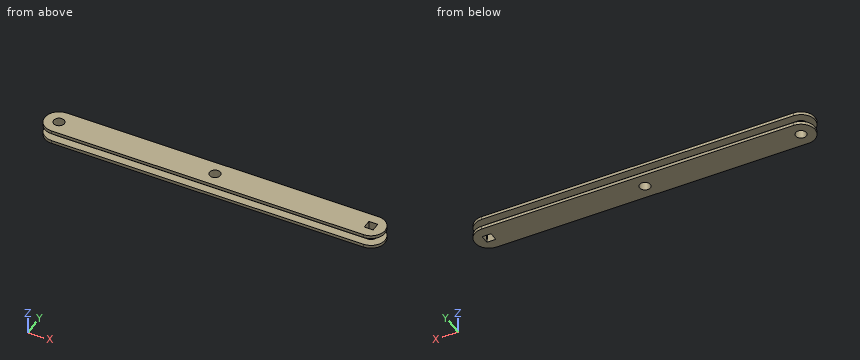
from build123d import *

# Parameters (mm, degrees)
ESQUISSE1_W             = 152.4
ESQUISSE1_H             = 12.7
BOSS_EXTRU_1_DEPTH      = 6.35
ESQUISSE2_W             = 3.967596046
ESQUISSE2_H             = 3.967596046
ESQUISSE2_W_2           = 3.367596046
ESQUISSE2_H_2           = 3.367596046
ESQUISSE2_W_3           = 3.167596046
ESQUISSE2_H_3           = 3.167596046
ESQUISSE2_R             = 2.38125
ENL_V_MAT_EXTRU_1_DEPTH = 154.060029074
SKETCH1_W               = 14.17076538
SKETCH1_H               = 3.495000122
CUT_REVOLVE1_ANGLE      = 180
SKETCH2_W               = 3.495000122
SKETCH2_H               = 3.683
CUT_EXTRUDE1_DEPTH      = 154.060029074
ESQUISSE2_3_W           = 3.367596046
ESQUISSE2_3_H           = 3.367596046
ESQUISSE2_3_W_2         = 3.167596046
ESQUISSE2_3_H_2         = 3.167596046
CUT_EXTRUDE2_DEPTH      = 154.060029074


with BuildPart() as part:
    # Esquisse1 → Boss.-Extru.1 (new body)
    with BuildSketch(Plane.XY):
        with Locations((-76.2, 6.35)):
            Rectangle(ESQUISSE1_W, ESQUISSE1_H)
    extrude(amount=-BOSS_EXTRU_1_DEPTH)

    # Esquisse2 → Enlèv. mat.-Extru.1 (cut, through all)
    # profile 1 of 8: a face of its own
    with BuildSketch(Plane.XY):
        with BuildLine():
            Line((0, 0), (0, 6.35))
            ThreePointArc((0, 6.35), (-1.859871939, 1.859871939), (-6.35, 0))
            Line((-6.35, 0), (0, 0))
        make_face()
    # profile 2 of 8: a face of its own
    with BuildSketch(Plane.XY):
        with BuildLine():
            Line((0, 12.7), (-6.35, 12.7))
            ThreePointArc((-6.35, 12.7), (-1.859871939, 10.840128061), (0, 6.35))
            Line((0, 6.35), (0, 12.7))
        make_face()
    # profile 3 of 8: a face of its own
    with BuildSketch(Plane.XY):
        with BuildLine():
            ThreePointArc((-152.4, 6.35), (-150.540128061, 10.840128061), (-146.05, 12.7))
            Line((-146.05, 12.7), (-152.4, 12.7))
            Line((-152.4, 12.7), (-152.4, 6.35))
        make_face()
    # profile 4 of 8: a face of its own
    with BuildSketch(Plane.XY):
        with BuildLine():
            ThreePointArc((-146.05, 0), (-150.540128061, 1.859871939), (-152.4, 6.35))
            Line((-152.4, 6.35), (-152.4, 0))
            Line((-152.4, 0), (-146.05, 0))
        make_face()
    # profile 5 of 8: a face of its own
    with BuildSketch(Plane.XY):
        with Locations((-6.35, 6.35)):
            Rectangle(ESQUISSE2_W, ESQUISSE2_H)
        with Locations((-6.35, 6.35)):
            Rectangle(ESQUISSE2_W_2, ESQUISSE2_H_2, mode=Mode.SUBTRACT)
    # profile 6 of 8: a face of its own
    with BuildSketch(Plane.XY):
        with Locations((-6.35, 6.35)):
            Rectangle(ESQUISSE2_W_3, ESQUISSE2_H_3)
    # profile 7 of 8: a face of its own
    with BuildSketch(Plane.XY):
        with Locations((-146.05, 6.35)):
            Circle(ESQUISSE2_R)
    # profile 8 of 8: a face of its own
    with BuildSketch(Plane.XY):
        with Locations((-76.2, 6.35)):
            Circle(ESQUISSE2_R)
    extrude(amount=-ENL_V_MAT_EXTRU_1_DEPTH, mode=Mode.SUBTRACT)


with BuildPart() as enl_v_mat_extru_1_piece_1:
    # of the separate pieces the step leaves, piece 1, a body of its own (enl_v_mat_extru_1_pieces)
    add(part.part.solids().sort_by_distance((-6.35, 0, 0))[0])

    # Sketch1 → Cut-Revolve1 (revolve, symmetric, cut)
    with BuildSketch(Plane(origin=(0, 6.35, 0), x_dir=(1, 0, 0), z_dir=(0, 1, 0))) as cut_revolve1_sk:
        Polygon((-150.5585, 1.427499939), (-152.4, 1.427499939), (-152.4, 4.922500061), (-150.5585, 4.922500061), (-148.717, 4.922500061), (-148.717, 1.427499939), align=None)
        with Locations((-159.48538269, 3.175)):
            Rectangle(SKETCH1_W, SKETCH1_H)
    cut_revolve1 = revolve(axis=Axis((-146.05, 6.35, -6.35), (0, 0, 1)), revolution_arc=CUT_REVOLVE1_ANGLE / 2, mode=Mode.SUBTRACT)
    cut_revolve1 = cut_revolve1 + revolve(cut_revolve1_sk.sketch, axis=Axis((-146.05, 6.35, -6.35), (0, 0, -1)), revolution_arc=CUT_REVOLVE1_ANGLE / 2, mode=Mode.SUBTRACT)

    # Mirror1: Cut-Revolve1 across plane
    add(cut_revolve1.mirror(Plane(origin=(-76.2, 0, 0), x_dir=(0, 0, 1), z_dir=(1, 0, 0))), mode=Mode.SUBTRACT)

    # Sketch2 → Cut-Extrude1 (cut, through all)
    with BuildSketch(Plane(origin=(0, 0, 0), x_dir=(0, 0, -1), z_dir=(1, 0, 0))):
        with Locations((3.175, 10.8585)):
            Rectangle(SKETCH2_W, SKETCH2_H)
    cut_extrude1 = extrude(amount=-CUT_EXTRUDE1_DEPTH, mode=Mode.SUBTRACT)

    # Mirror2: Cut-Extrude1 across plane
    add(cut_extrude1.mirror(Plane.ZX.offset(6.35)), mode=Mode.SUBTRACT)


with BuildPart() as enl_v_mat_extru_1_piece_2:
    # of the separate pieces the step leaves, piece 2, a body of its own (enl_v_mat_extru_1_pieces)
    add(part.part.solids().sort_by_distance((-8.033798023, 4.666201977, 0))[0])

    # Esquisse2<3> → Cut-Extrude2 (cut, through all)
    with BuildSketch(Plane.XY):
        with Locations((-6.35, 6.35)):
            Rectangle(ESQUISSE2_3_W, ESQUISSE2_3_H)
        with Locations((-6.35, 6.35)):
            Rectangle(ESQUISSE2_3_W_2, ESQUISSE2_3_H_2, mode=Mode.SUBTRACT)
    extrude(amount=-CUT_EXTRUDE2_DEPTH, mode=Mode.SUBTRACT)


solid = enl_v_mat_extru_1_piece_1.part
Could you check a few things on this model? Use its own coordinates, in mm. Give positions to 0.01 mm unless a question says otherwise; leave off trailing zeros. Order: outer loops, then holes, each group sorted by start corner. A loop starts at its lowest first (then second) coordinate and runs counter-clockwise, first axis right, second up. Notation, with made-up numbers: (-5.75, 9) - (52.25, 9) arc R28 ccw to (52.25, 44) - close; hole circle Ø4 at (53.5, 75). An arc over 180 degrees is marked (long way). One line per item, written item: value. Start each with the question number.
1. Imagine slicing it at C-C on x = -42. List the corners of the cut face in (y, z) for me.
2. Imagine slicing it at B-B on x = -76.2. List the corners of the cut face in (y, z) for me.
3. If I drill on probe 1 along Z at (x, y) = (-26.5, 12.25); probe 2 along Y at (x, z) = (-76.2, -2.75); probe 3 along X at (y, z) = (5.75, -3.75), over which ranges is the centre line in solid material (lowest first)?
4. For P1, Ø1.5, axis at y = 2.5, z = -1, coming from the -X side; P2, Ø3, axis at x = -146.05, y = 6.35, coming from the +Z side (3 decimals); P3, Ø1.5, axis at x = -116, z = -4, coming from the +Y side; P4, Ø1.7, axis at x = -74.5, z = -3, coming from the -Y side, each with a flat end and sliding along its axis, tell me the tip position at first contact or that it passes through.
5. Imagine slicing it at A-A on z = -2.75. List the corners of the cut face in (x, y) for me, plus the area to 3 significant figures.
Values:
1. outline: (0, -6.35) - (12.7, -6.35) - (12.7, -4.92) - (9.02, -4.92) - (9.02, -1.43) - (12.7, -1.43) - (12.7, 0) - (0, 0) - (0, -1.43) - (3.68, -1.43) - (3.68, -4.92) - (0, -4.92) - close
2. outline: (0, -6.35) - (3.97, -6.35) - (3.97, 0) - (0, 0) - (0, -1.43) - (3.68, -1.43) - (3.68, -4.92) - (0, -4.92) - close; (8.73, -6.35) - (12.7, -6.35) - (12.7, -4.92) - (9.02, -4.92) - (9.02, -1.43) - (12.7, -1.43) - (12.7, 0) - (8.73, 0) - close
3. probe 1: -6.35 to -4.92, -1.43 to 0
3. probe 2: 3.68 to 3.97, 8.73 to 9.02
3. probe 3: -148.65 to -148.35, -143.75 to -78.5, -73.9 to -8.33, -4.37 to -3.75
4. P1: x = -151.59
4. P2: through
4. P3: y = 9.02
4. P4: y = 3.68
5. outline: (-146.05, 3.68) - (-6.35, 3.68) arc R2.67 ccw to (-4.57, 4.37) - (-8.33, 4.37) - (-8.33, 8.33) - (-4.57, 8.33) arc R2.67 ccw to (-6.35, 9.02) - (-146.05, 9.02) arc R2.67 ccw to start; (-4.37, 4.57) arc R2.67 ccw to (-4.37, 8.13) - close; hole circle Ø4.76 at (-146.05, 6.35); hole circle Ø4.76 at (-76.2, 6.35)
5. area: 716 mm²
